from build123d import *

# Parameters (mm, degrees)
SKETCH2_W           = 123.41
SKETCH2_H           = 71.848
SKETCH2_R           = 1.360904611
SKETCH2_R_2         = 1.6
SKETCH2_W_2         = 2.132357215
SKETCH2_H_2         = 23.848
SKETCH2_W_3         = 45.41
SKETCH2_H_3         = 1.677202247
SKETCH2_W_4         = 1.620785214
SKETCH2_H_4         = 1.892776038
BOSS_EXTRUDE1_DEPTH = 2


with BuildPart() as part:
    # Sketch2 → Boss-Extrude1 (new body)
    with BuildSketch(Plane(origin=(0, 0, 0), x_dir=(1, 0, 0), z_dir=(0, 1, 0))):
        with Locations((56.450952339, 30.702122774)):
            Rectangle(SKETCH2_W, SKETCH2_H)
        with Locations(Location((3.77654317, 3.778122774, 0), (0, 0, 270))):
            Circle(SKETCH2_R, mode=Mode.SUBTRACT)
        with Locations(Location((109.18654317, 3.778122774, 0), (0, 0, 270))):
            Circle(SKETCH2_R, mode=Mode.SUBTRACT)
        with Locations(Location((3.77654317, 57.626122774, 0), (0, 0, 270))):
            Circle(SKETCH2_R_2, mode=Mode.SUBTRACT)
        with Locations(Location((109.18654317, 57.626122774, 0), (0, 0, 270))):
            Circle(SKETCH2_R, mode=Mode.SUBTRACT)
        with Locations((-2.289635438, 30.702122774)):
            Rectangle(SKETCH2_W_2, SKETCH2_H_2, mode=Mode.SUBTRACT)
        with Locations((56.48154317, 63.464723898)):
            Rectangle(SKETCH2_W_3, SKETCH2_H_3, mode=Mode.SUBTRACT)
        with Locations((114.996935777, 30.702122774)):
            Rectangle(SKETCH2_W_4, SKETCH2_H_2, mode=Mode.SUBTRACT)
        with Locations((56.48154317, -2.168265245)):
            Rectangle(SKETCH2_W_3, SKETCH2_H_4, mode=Mode.SUBTRACT)
    extrude(amount=BOSS_EXTRUDE1_DEPTH)


solid = part.part
Geometry check sheet. Reference: the model listing, model coordinates, mm. Give positions to 0.01 mm unless a question says otherwise; leave off trailing zeros. Loops run counter-clockwise (first coordinate to the right, second up) from the corner with the lowest first, then second, coordinate; pieces in that order, holes last. Notation, with made-up numbers: M 25.5,12.25 L 57.5,12.25 A24 ccw 57.5,37.25 Z; hole C 85,87 d2. An arc over 180 degrees is marked long. Write each question's results on one line, items separated by ' | '.
1) Release check for a two-part mould opening along Z. For faces 1 (the face through (56, 0, -31)), 2 (the face through (4.26, 0.99, -56.1)) record: +Z half, -Z half, draft (parallel to the pull), parting line (faces both ways), or undercut.
Answers follow:
face 1: draft | face 2: undercut
2) Section check B-B, the plane z = -27. Record the boundary of the cut face in (x, y), plus the area to 3 significant figures.
Answers follow:
outline: M -5.25,0 L -3.36,0 L -3.36,2 L -5.25,2 Z; M -1.22,0 L 114.19,0 L 114.19,2 L -1.22,2 Z; M 115.81,0 L 118.16,0 L 118.16,2 L 115.81,2 Z | area: 239 mm2
3) Gauge pin test, flat end, axial feed: pin 1 (10 mm diameter, centred on x = 99.5, z = -48.5, fed in from -Y). Record the tip position at first contact, or that the pin passes through.
Answers follow:
pin 1: y = 0
4) Section check C-C, the plane y = 0.7. Count the separate pieces of the cut face and the enclosed holes in it, plus the area to 3 significant figures.
Answers follow:
separate pieces: 1 | enclosed holes: 8 | area: 8,590 mm2
5) Section check A-A, the plane x = 36. Record the boundary of the cut face in (y, z).
Answers follow:
outline: M 0,-66.63 L 2,-66.63 L 2,-64.3 L 0,-64.3 Z; M 0,-62.63 L 2,-62.63 L 2,1.22 L 0,1.22 Z; M 0,3.11 L 2,3.11 L 2,5.22 L 0,5.22 Z
6) Thickness scan on line 1 (Z direction, x = 67, y = 1); line 2 (X direction, y = 1.65, z = -22.5). Record the ranges inside material, lowest first.
Answers follow:
line 1: -66.63 to -64.3, -62.63 to 1.22, 3.11 to 5.22 | line 2: -5.25 to -3.36, -1.22 to 114.19, 115.81 to 118.16
